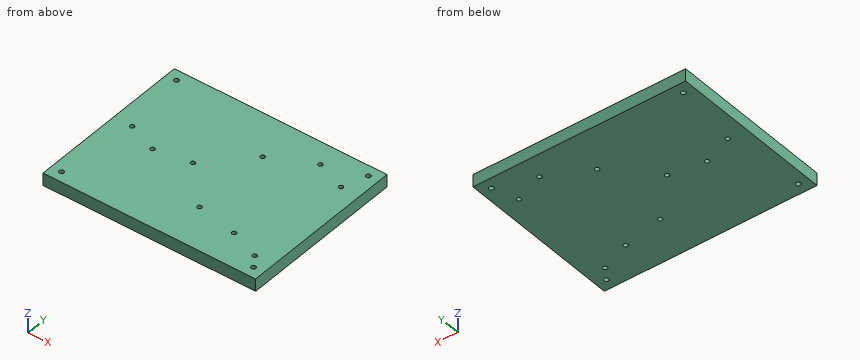
```python
from build123d import *

# Parameters (mm, degrees)
SKETCH_W        = 205
SKETCH_H        = 160
PAD_DEPTH       = 12
SKETCH001_R     = 2.1
POCKET_DEPTH    = 12.001
SKETCH002_R     = 2.25
POCKET001_DEPTH = 12.001


with BuildPart() as part:
    # Sketch → Pad (new body)
    with BuildSketch(Plane.XY):
        Rectangle(SKETCH_W, SKETCH_H)
    extrude(amount=PAD_DEPTH)

    # Sketch001 → Pocket (cut, through all)
    with BuildSketch(Plane.XY.offset(12)):
        with Locations((-84.525, 5.829)):
            Circle(SKETCH001_R)
        with Locations((-55.475, -5.83)):
            Circle(SKETCH001_R)
        with Locations((-21.275, 0)):
            Circle(SKETCH001_R)
        with Locations((15.575, 38.42)):
            Circle(SKETCH001_R)
        with Locations((15.575, -38.42)):
            Circle(SKETCH001_R)
        with Locations((55.475, 58.3295)):
            Circle(SKETCH001_R)
        with Locations((84.525, 46.6705)):
            Circle(SKETCH001_R)
        with Locations((55.475, -46.6705)):
            Circle(SKETCH001_R)
        with Locations((84.525, -58.3295)):
            Circle(SKETCH001_R)
    extrude(amount=-POCKET_DEPTH, mode=Mode.SUBTRACT)

    # Sketch002 → Pocket001 (cut, through all)
    with BuildSketch(Plane.XY.offset(12)):
        with Locations((-92.5, 70)):
            Circle(SKETCH002_R)
        with Locations((92.5, 70)):
            Circle(SKETCH002_R)
        with Locations((-92.5, -70)):
            Circle(SKETCH002_R)
        with Locations((92.5, -70)):
            Circle(SKETCH002_R)
    extrude(amount=-POCKET001_DEPTH, mode=Mode.SUBTRACT)


solid = part.part
```
Read the model definition and answer for the solid it produces. Units are mm, in the model's axes. Give positions to 0.01 mm unless a question says otherwise; leave off trailing zeros. Write each loop counter-clockwise with the first axis right and the second up, starting at its lowest first coordinate (ties: lowest second). Pieces come first, ordered by that corner, then holes. Notation, with made-up numbers: M 49,-28.5 L 103,-28.5 A19 cw 103,-11.5 Z; hole C -14,-21 d2. An arc over 180 degrees is marked long. Put each result on its own line as item: value. Start each with the question number.
1. Consider line 1 along Y through (x, z) = (-92.5, 8.75); line 2 along X through (y, z) = (-71, 4.75); line 3 along Y through (x, z) = (14, 1). Determine where each line is inside the solid, lowest interval first.
2. The part is cut by section B-B, the plane x = 92.5. Give the vertices of the cut face in (y, z).
3. The part is cut by section A-A, the plane y = -38.42. Give the vertices of the cut face in (x, z) (3 decimals).
4. This flat-tipped pin is pushed along its axis until it touches: pin 1 Ø2.5 at (x, y) = (-84.525, 5.829) entering from +Z. Where does it stop, or does it pass through?
Final values:
1. line 1: y = -80 to -72.25, -67.75 to 67.75, 72.25 to 80
1. line 2: x = -102.5 to -94.52, -90.48 to 90.48, 94.52 to 102.5
1. line 3: y = -80 to -39.81, -37.03 to 37.03, 39.81 to 80
2. outline: M -80,0 L -72.25,0 L -72.25,12 L -80,12 Z; M -67.75,0 L 67.75,0 L 67.75,12 L -67.75,12 Z; M 72.25,0 L 80,0 L 80,12 L 72.25,12 Z
3. outline: M -102.5,0 L 13.475,0 L 13.475,12 L -102.5,12 Z; M 17.675,0 L 102.5,0 L 102.5,12 L 17.675,12 Z
4. pin 1: passes through
